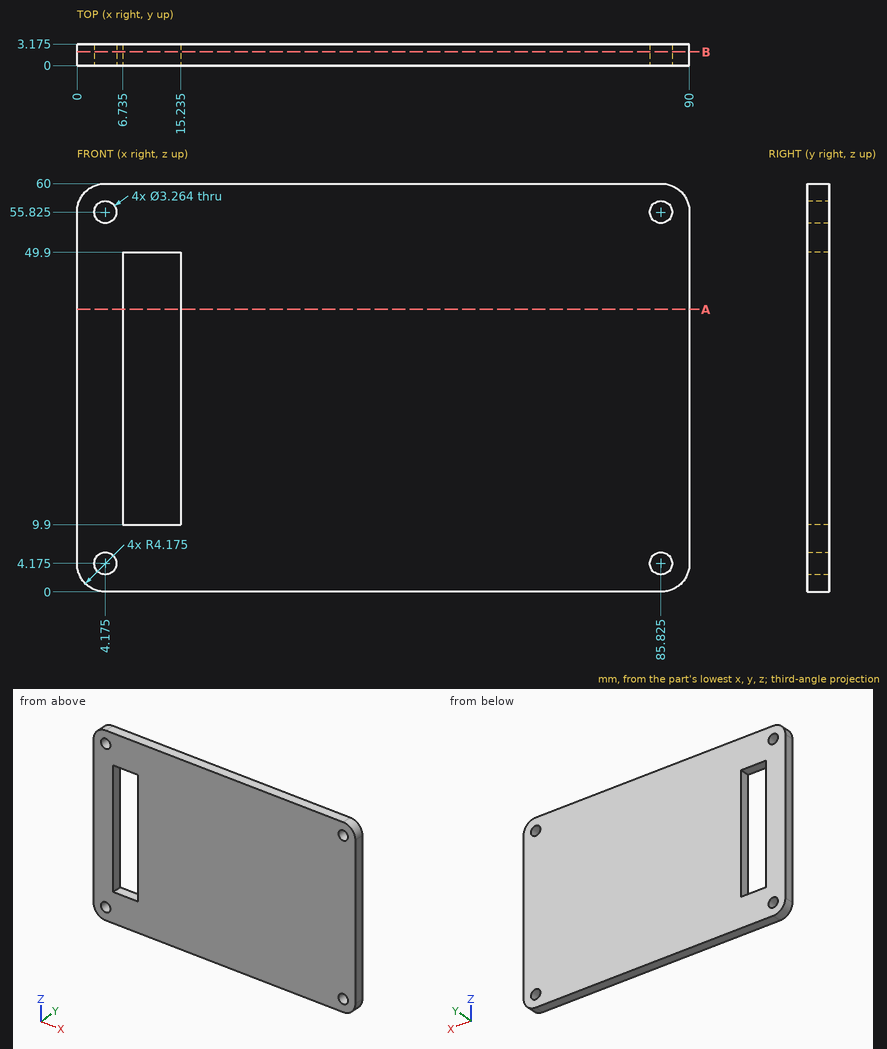
Geometry: see drawing. Coordinates: mm, zero at the bounding-box minimum. Coordinates: 2 decimals unless noted, no trailing zeros. Order: outer loops, then holes, each group sorted by start corner. A loop starts at its lowest first (then second) coordinate and runs counter-clockwise, first axis right, second up. Notation, with made-up numbers: M 79,59.25 L 123,59.25 A22 ccw 123,66.25 Z; hole C 5.5,2.5 d2. An arc over 180 degrees is marked long. Answer in a Markdown table with one row per item. Add a question column.
Q1. Section query B-B on y = 2. Count the separate pieces of the cut face and the enclosed holes in it, and give its area (3 significant figures).
Q2. Line query: L1, parallel to X at y = 2.85, z = 31 (1 decimal); L2, parallel to Z at x = 13.5, y = 2.55; L3, parallel to X at y = 1.55, z = 3. Output: solid intervals per line, ascending.
Q3. Contact query for a flat-ended pin moving along its axis: P1, Ø2, axis at x = 4.175, z = 4.175, coming from the +Y side. Output: stop coordinate, or through.
Q4. Section query A-A on z = 41.5. Return the cut outline in (x, y) (1 decimal), and give its area (3 significant figures).
Completed:
| question | item | result |
|---|---|---|
| 1 | separate pieces | 1 |
| 1 | enclosed holes | 5 |
| 1 | area | 5,010 mm2 |
| 2 | L1 | x = 0 to 6.7, 15.2 to 90 |
| 2 | L2 | z = 0 to 9.9, 49.9 to 60 |
| 2 | L3 | x = 0.17 to 3.04, 5.31 to 84.69, 86.96 to 89.83 |
| 3 | P1 | passes through |
| 4 | outline | M 0,0 L 6.7,0 L 6.7,3.2 L 0,3.2 Z; M 15.2,0 L 90,0 L 90,3.2 L 15.2,3.2 Z |
| 4 | area | 259 mm2 |
